from build123d import *

# Parameters (mm, degrees)
BOSS_EXTRUDE1_DEPTH = 7
SKETCH2_W           = 4.25
SKETCH2_H           = 7
BOSS_EXTRUDE2_DEPTH = 8
SKETCH3_R           = 1.899478465
SKETCH3_R_2         = 1.75
CUT_EXTRUDE1_DEPTH  = 19


with BuildPart() as part:
    # Sketch1 → Boss-Extrude1 (new body)
    with BuildSketch(Plane(origin=(0, 0, 0), x_dir=(1, 0, 0), z_dir=(0, 1, 0))):
        Polygon((6.25, 0), (19.75, 0), (19.75, 7.2), (26, 7.2), (26, 14.2), (0, 14.2), (0, 7.2), (6.25, 7.2), align=None)
    extrude(amount=BOSS_EXTRUDE1_DEPTH)

    # Sketch2 → Boss-Extrude2 (add)
    with BuildSketch(Plane(origin=(0, 7, 0), x_dir=(1, 0, 0), z_dir=(0, 1, 0))):
        with Locations((8.375, 10.7)):
            Rectangle(SKETCH2_W, SKETCH2_H)
        with Locations((17.625, 10.7)):
            Rectangle(SKETCH2_W, SKETCH2_H)
    extrude(amount=BOSS_EXTRUDE2_DEPTH)

    # Sketch3 → Cut-Extrude1 (cut)
    with BuildSketch(Plane(origin=(0, 7, 0), x_dir=(1, 0, 0), z_dir=(0, 1, 0))):
        with Locations(Location((22.75, 10.7, 0), (0, 0, 270))):
            Circle(SKETCH3_R)
        with Locations(Location((3.25, 10.7, 0), (0, 0, 270))):
            Circle(SKETCH3_R_2)
    extrude(amount=-CUT_EXTRUDE1_DEPTH, mode=Mode.SUBTRACT)


solid = part.part
Can you work these out from the model? Positions are in its coordinate system, mm. A direction names the side the tool comes from. Coordinates: 2 decimals unless noted, no trailing zeros. Loops run counter-clockwise (first coordinate to the right, second up) from the corner with the lowest first, then second, coordinate; pieces in that order, holes last. Notation, with made-up numbers: M -17,-18.5 L 42,-18.5 A20 cw 42,9.5 Z; hole C 16.5,-26.5 d9. An arc over 180 degrees is marked long. Return JSON: item names as keys, results as strings. Group by question number.
Item 1: On a 3-axis mill with a long thin cutter (end or side, diameter ignored), from which of +Z, -Z, +X, -X, +Y, -Y can I reach the whole of each face in a straight line? I mean faces 1 (the flat face through (6.25, 11, -11)), 2 (the flat face through (19.75, 3, -4)), 3 (the flat face through (3, 3, -7.2)). Say none if no direction works.
Item 2: I'm going to push flat-ended pins straight in: pin 1 Ø4 at (y, z) = (3, -2) entering from +X; pin 2 Ø3.5 at (x, y) = (16.5, 10.5) entering from +Z; pin 3 Ø5 at (x, z) = (2, -9) entering from +Y; pin 4 Ø5.5 at (y, z) = (9.5, -9.5) entering from -X. Where does each tip first touch, or does it pass through?
Item 3: Imagine slicing it at B-B (z = -10.7). Please give me the cut outline in (x, y).
Item 4: Imagine slicing it at D-D (x = 22.75). Please give me the cut outline in (y, z).
Item 5: Imagine slicing it at C-C (y = 5). Please give me the cut outline in (x, z).
Item 6: Imagine slicing it at A-A (x = 3.25). Please give me the cut outline in (y, z).
Item 7: If I drill on L1, parallel to X at y = 2.25, z = -10.7; L2, parallel to X at y = 7.25, z = -13.25; L3, parallel to Y at x = 3.5, z = -8, over which ranges is the centre line in solid material (lowest first)? Write a range as from..to.
Item 8: Thinking about a two-plate mould opening in Z: for faces 4 (the flat face through (13, 6, -14.2)), 5 (the flat face through (6.25, 3, -4)), 6 (the flat face through (13, 3, 0)), 7 (the cylindrical face through (23.32, 3.55, -8.89)), which applies, released by +Z, released by -Z, zero draft, split by the parting line, or undercut?
Verdict:
{
 "1": {"face 1": "+Z, -Z, -X, +Y", "face 2": "+Z, +X, +Y, -Y", "face 3": "+Z, -X, +Y, -Y"},
 "2": {"pin 1": "stops at x = 19.75", "pin 2": "stops at z = -7.2", "pin 3": "stops at y = 7", "pin 4": "stops at x = 0"},
 "3": {"outline": "M 0,0 L 1.5,0 L 1.5,7 L 0,7 Z; M 5,0 L 20.85,0 L 20.85,7 L 19.75,7 L 19.75,15 L 15.5,15 L 15.5,7 L 10.5,7 L 10.5,15 L 6.25,15 L 6.25,7 L 5,7 Z; M 24.65,0 L 26,0 L 26,7 L 24.65,7 Z"},
 "4": {"outline": "M 0,-14.2 L 7,-14.2 L 7,-12.6 L 0,-12.6 Z; M 0,-8.8 L 7,-8.8 L 7,-7.2 L 0,-7.2 Z"},
 "5": {"outline": "M 0,-14.2 L 26,-14.2 L 26,-7.2 L 19.75,-7.2 L 19.75,0 L 6.25,0 L 6.25,-7.2 L 0,-7.2 Z; hole C 3.25,-10.7 d3.5; hole C 22.75,-10.7 d3.8"},
 "6": {"outline": "M 0,-14.2 L 7,-14.2 L 7,-12.45 L 0,-12.45 Z; M 0,-8.95 L 7,-8.95 L 7,-7.2 L 0,-7.2 Z"},
 "7": {"L1": "x = 0..1.5, 5..20.85, 24.65..26", "L2": "x = 6.25..10.5, 15.5..19.75", "L3": "y = 0..7"},
 "8": {"face 4": "released by -Z", "face 5": "zero draft", "face 6": "released by +Z", "face 7": "undercut"}
}
